Verification items for the finished model (mm, model axes). A direction names the side the tool comes from. Round coordinates to 2 decimals unless told otherwise and drop trailing zeros. Order: outer loops, then holes, each group sorted by start corner. A loop starts at its lowest first (then second) coordinate and runs counter-clockwise, first axis right, second up. Notation, with made-up numbers: M 54,75.5 L 74,75.5 A17 ccw 74,108.5 Z; hole C 25.5,-8.75 d3. An arc over 180 degrees is marked long. Write item = value, one per line. Start each with the question number.
Autodesk Inventor part; units mm, degrees
ref_plane "Arbeitsebene1" through (0, 0, 3) normal (0, 0, 1) x (1, 0, 0)
ref_plane "YZ Plane" through (0, 0, 0) normal (1, 0, 0) x (0, 1, 0)
ref_plane "XZ Plane" through (0, 0, 0) normal (0, 1, 0) x (-1, 0, 0)
sketch "Skizze1" plane through (0, 0, 0) normal (0, 0, 1) x (1, 0, 0)
  line L0 (-2.5, 0) -> (5.5, 0)
  line L1 (9.5, 2.5) -> (9.5, 4)
  line L2 (9.5, 4) -> (2, 4)
  line L3 (-2.5, 2.5) -> (-2.5, 5.5)
  line L4 (-2.5, 5.5) -> (0, 5.5)
  line L5 (2, 4) -> (1.3045, 3.8136)
  line L6 (1.2009, 3.8) -> (0.3, 3.8)
  line L7 (-0.0913, 4.2832) -> (0, 4.7125)
  line L8 (0, 4.7125) -> (0, 5.5)
  arc A0 (-0.0913, 4.2832) -> (0.3, 3.8) centre (0.3, 4.2) ccw
  arc A1 (1.2009, 3.8) -> (1.3045, 3.8136) centre (1.2009, 4.2) ccw
  line L9 (-4.9, 0) -> (11.9, 0)
  line L10 (0, -0.9) -> (0, 5.4)
  line L11 (-2.5, 2.5) -> (9.5, 2.5)
  dimension "d0" = 11
  dimension "d1" = 8
  dimension "d2" = 12
  dimension "d3" = 12
  dimension "d4" = 0.4
  dimension "d5" = 0.1
  dimension "d6" = 2
  dimension "d7" = 15
  dimension "d8" = 0.2
  dimension "d9" = 0.4
  dimension "d10" = 2.5
  dimension "d11" = 5
revolve "Körper" add sketch "Skizze1" angle 360 about axis through (-2.5, 0, 0) along (1, 0, 0) contours L11 L10 A0 L6 A1 L5 L2 L1 | L11 L3 L4 L8 L7 A0 L10
chamfer "Fase1" distance 1 angle 15 1 edges at (9.5, -4, 0) measured on face at (7, 3.9482, -0.6416)
fillet "Rundung1" radius 1 1 edges at (-2.5, -2.5, 0)
ref_plane "Arbeitsebene1" through (0, 0, 3) normal (0, 0, 1) x (1, 0, 0)
sketch "Skizze2" plane through (0, 0, 3) normal (0, 0, 1) x (1, 0, 0)
  line L0 (9.5, 3.7321) -> (9.5, -3.7321)
  line L1 (-2.5, -5.5) -> (-2.5, 5.5)
  point P0 (0, 0)
  point P1 (3.5, 0)
  point P2 (9.5, 0)
  dimension "d39" = 6
hole "Bohrung1" at (3.5, 0, 3) direction (0, 0, -1) diameter 0.5 end through all both
equation "\"d12\" = PHH"
equation "\"d13\" = ANG"
equation "\"d29\" = PHH"
equation "\"d14\" = RR"
equation "\"d0\" = KOD"
equation "\"d1\" = SD2"
equation "\"d2\" = NLG"
equation "\"d4\" = FSRR"
equation "\"d5\" = FST2"
equation "\"d6\" = FSB"
equation "\"d8\" = FST1"
equation "\"d9\" = FSRR"
equation "\"d10\" = KOH"
equation "\"d11\" = NND"
equation "\"NLG\" = 12"
equation "\"NND\" = 5"
equation "\"KOD\" = 11"
equation "\"KOH\" = 2.5"
equation "\"SD2\" = 8"
equation "\"FST1\" = 0.2"
equation "\"FST2\" = 0.1"
equation "\"FSB\" = 2"
equation "\"FSRR\" = 0.4"
equation "\"PHH\" = 1"
equation "\"ANG\" = 15deg"
equation "\"RR\" = 1"
equation "\"NNDMIN\" = 4.1"
equation "\"FSH\" = 1.1"
equation "\"NNDMAX\" = 5"
equation "\"SEWI\" = 30deg"
properties part number "DIN 172 - A 5 x 12" material "Stahl, weich"
1) Access from +Z, -Z, +X, -X, +Y, -Y to the whole of each face (thin tool, end or side, straight path). Record for faces 4 (the cylindrical face through (-1.23, -1.19, -5.37)), 5 (the cylindrical face through (0.744, -3.796, -0.167)).
2) Release check for a two-part mould opening along Z. For faces 1 (the cylindrical face through (4.08, -0.54, -2.44)), 2 (the flat face through (-2.5, 4, 0)), 3 (the cylindrical face through (5.204, -0.867, 3.905)) record: pulls with the +Z half, pulls with the -Z half, needs draft (parallel to the pull), parting line crosses it, or undercut.
3) Cross-section at A-A, the plane z = 0. Enter the section's corners in (x, y), then the cut area to 3 significant figures.
4) Cross-section at B-B, the plane y = 0. Give the number of separate pieces and of enclosed holes in the cut face, then the cut area to 3 significant figures.
5) Scan lines: probe 1 along X at (y, z) = (0, -3.55); probe 2 along Z at (x, y) = (5.5, 0); probe 3 along Y at (x, z) = (1.5, -0.5). Record each from-to range of solid material in increasing order.
6) Gauge pin test, flat ends, axial feed: P1, Ø2, axis at x = 7, z = -4, coming from the -Y side; P2, Ø4, axis at x = 3, y = 1.5, coming from the -Z side; P3, Ø1, axis at x = 2, z = 1.5, coming from the +Y side; P4, Ø2, axis at y = 0.5, z = 3, coming from the -X side. Record the tip position at first contact, or that the pin passes through.
7) Cross-section at D-D, the plane x = 1. Enter the section's corners in (y, z), then the cut area to 3 significant figures.
Geometry results:
q1.face_4 = +X, -X
q1.face_5 = none
q2.face_1 = undercut
q2.face_2 = needs draft
q2.face_3 = parting line crosses it
q3.outline = M -2.5,-5.5 L 0,-5.5 L 0,-4.71 L -0.09,-4.28 A0.4 cw 0.3,-3.8 L 1.2,-3.8 A0.4 cw 1.3,-3.81 L 2,-4 L 8.5,-4 L 9.5,-3.73 L 9.5,-2.5 L -1.5,-2.5 A1 ccw -2.5,-3.5 Z; M -2.5,3.5 A1 ccw -1.5,2.5 L 9.5,2.5 L 9.5,3.73 L 8.5,4 L 2,4 L 1.3,3.81 A0.4 cw 1.2,3.8 L 0.3,3.8 A0.4 cw -0.09,4.28 L 0,4.71 L 0,5.5 L -2.5,5.5 Z
q3.area = 42.1 mm^2
q4.separate_pieces = 4
q4.enclosed_holes = 0
q4.area = 40.6 mm^2
q5.probe_1 = -2.5 to 3.25, 3.75 to 9.5
q5.probe_2 = -4 to -2.5, 2.5 to 4
q5.probe_3 = -3.83 to -2.45, 2.45 to 3.83
q6.P1 = -2.65
q6.P2 = -4
q6.P3 = 3.87
q6.P4 = -2.5
q7.outline = C 0,0 d7.6; hole C 0,0 d5
q7.area = 25.7 mm^2
